```python
from build123d import *

# Parameters (mm, degrees)
F0_R           = 31.75
F1_DEPTH       = 10.16
F2_W           = 25.4
F2_H           = 24.13
F3_DEPTH       = 19.05
F5_D           = 6.6
F5_CBORE_D     = 11.25
F5_CBORE_DEPTH = 5
F7_D           = 7.1374


with BuildPart() as f1:
    # F0 (on Top) → F1 (new body)
    with BuildSketch(Plane.XY):
        Circle(F0_R)
    extrude(amount=F1_DEPTH)

    # F2 (on face) → F3 (join)
    with BuildSketch(Plane.XY.offset(10.16)):
        Rectangle(F2_W, F2_H)
    extrude(amount=F3_DEPTH)

    # F5 (through all)
    with Locations(Plane.XY.offset(10.16)):
        with Locations((-17.6911045585, 17.6911045585), (17.6911045585, 17.6911045585), (-17.6911045585, -17.6911045585), (17.6911045585, -17.6911045585)):
            CounterBoreHole(F5_D / 2, F5_CBORE_D / 2, F5_CBORE_DEPTH)

    # F7 (through all)
    with Locations(Plane.XZ.offset(12.065)):
        with Locations((0, 19.685)):
            Hole(F7_D / 2)


solid = f1.part
```
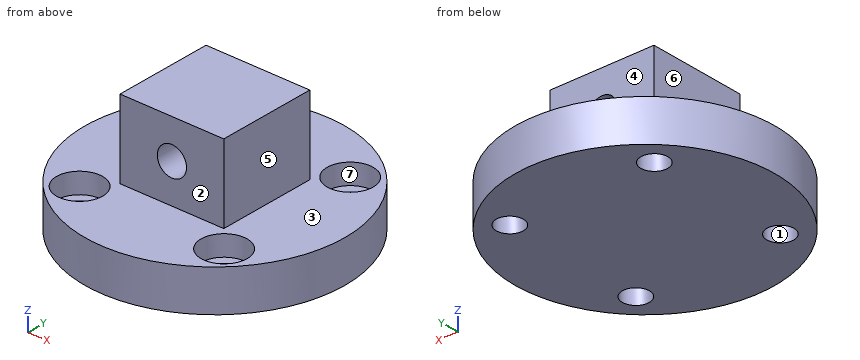
Work out the finished part from the listing and answer in its coordinate system (mm). Face numbers are marked on the shaded views. A direction names the side the tool comes from. Give positions to 0.01 mm unless a question says otherwise; leave off trailing zeros. Order: outer loops, then holes, each group sorted by start corner. A loop starts at its lowest first (then second) coordinate and runs counter-clockwise, first axis right, second up. Notation, with made-up numbers: (5.25, 51) -> (64.25, 51) arc R17 cw to (64.25, 76) -> close; hole circle Ø1 at (-10.75, 2). An arc over 180 degrees is marked (long way). Answer as CSV lines item,"result". Start each with the question number.
(1) Section B-B, the plane y = 0 is taken. Write down the section's boundary in (x, z) (3 decimals), plus the area to 3 significant figures.
(2) Section A-A, the plane x = 0 is taken. Write down the section's boundary in (y, z) (3 decimals), plus the area to 3 significant figures.
(3) Each of these flat-tipped pins is pushed along its axis until it touches: pin 1 Ø3 at (y, z) = (-18, 3.5) entering from +X; pin 2 Ø5 at (x, y) = (-22, -8) entering from +Z; pin 3 Ø5.5 at (y, z) = (5.5, 17.5) entering from +X. Where does it stop, or does it pass through?
(4) For a pull along Y with two mould halves and no side action, classify the marked faces 1, 2, 3 and 4 as released by +Y, released by -Y, zero draft, split by the parting line, or undercut.
(5) Section D-D, the plane y = -19.5 is taken. Write down the section's boundary in (x, z), plus the area to 3 significant figures.
(6) Section C-C, the plane x = -16.5 is taken. Write down the section's boundary in (y, z).
(7) Which of the six approach directions +Z, -Z, +X, -X, +Y, -Y give full straight-line access (tool end or side, diameter ignored) to the marked faces 5, 6 and 7?
(8) Consider line 1 along Y through (x, z) = (-18.5, 5.25); line 2 along X through (y, z) = (-10.5, 27.75); line 3 along X through (y, z) = (-8, 19). Determine where each line is inside the solid, lowest interval first.
Entries:
1,outline,"(-31.75, 0) -> (31.75, 0) -> (31.75, 10.16) -> (12.7, 10.16) -> (12.7, 29.21) -> (-12.7, 29.21) -> (-12.7, 10.16) -> (-31.75, 10.16) -> close; hole circle Ø7.137 at (0, 19.685)"
1,area,"1,090 mm²"
2,outline,"(-31.75, 0) -> (31.75, 0) -> (31.75, 10.16) -> (12.065, 10.16) -> (12.065, 16.116) -> (-12.065, 16.116) -> (-12.065, 10.16) -> (-31.75, 10.16) -> close; (-12.065, 23.254) -> (12.065, 23.254) -> (12.065, 29.21) -> (-12.065, 29.21) -> close"
2,area,"933 mm²"
3,pin 1,"x = 27.13"
3,pin 2,"z = 10.16"
3,pin 3,"x = 12.7"
4,face 1,"undercut"
4,face 2,"released by -Y"
4,face 3,"zero draft"
4,face 4,"released by +Y"
5,outline,"(-25.06, 0) -> (-20.45, 0) -> (-20.45, 5.16) -> (-23.02, 5.16) -> (-23.02, 10.16) -> (-25.06, 10.16) -> close; (-14.93, 0) -> (14.93, 0) -> (14.93, 5.16) -> (12.36, 5.16) -> (12.36, 10.16) -> (-12.36, 10.16) -> (-12.36, 5.16) -> (-14.93, 5.16) -> close; (20.45, 0) -> (25.06, 0) -> (25.06, 10.16) -> (23.02, 10.16) -> (23.02, 5.16) -> (20.45, 5.16) -> close"
5,area,"346 mm²"
6,outline,"(-27.13, 0) -> (-20.77, 0) -> (-20.77, 5.16) -> (-23.19, 5.16) -> (-23.19, 10.16) -> (-27.13, 10.16) -> close; (-14.61, 0) -> (14.61, 0) -> (14.61, 5.16) -> (12.19, 5.16) -> (12.19, 10.16) -> (-12.19, 10.16) -> (-12.19, 5.16) -> (-14.61, 5.16) -> close; (20.77, 0) -> (27.13, 0) -> (27.13, 10.16) -> (23.19, 10.16) -> (23.19, 5.16) -> (20.77, 5.16) -> close"
7,face 5,"+Z, +X, +Y, -Y"
7,face 6,"+Z, -X, +Y, -Y"
7,face 7,"+Z"
8,line 1,"-25.8 to -23.26, -12.12 to 12.12, 23.26 to 25.8"
8,line 2,"-12.7 to 12.7"
8,line 3,"-12.7 to -3.5, 3.5 to 12.7"
